from build123d import *

# Parameters (mm, degrees)
F0_W     = 1.7
F0_H     = 14.3
F3_D     = 11
F3_DEPTH = 80
F3_TIP   = 3.3047334047
F5_D     = 11
F5_DEPTH = 80
F5_TIP   = 3.3047334047


with BuildPart() as f1:
    # F0 (on Front) → F1 (revolve)
    with BuildSketch(Plane.XZ):
        Polygon((534, 14.3), (534, 0), (540, 0), (540, 15), (534, 15), align=None)
        with Locations((533.15, 7.15)):
            Rectangle(F0_W, F0_H)
        Polygon((0, 15), (0, 0), (532.3, 0), (532.3, 14.3), (532.3, 15), align=None)
        Polygon((-532.3, 15), (-532.3, 14.3), (-532.3, 0), (0, 0), (0, 15), align=None)
        with Locations((-533.15, 7.15)):
            Rectangle(F0_W, F0_H)
        Polygon((-534, 15), (-540, 15), (-540, 0), (-534, 0), (-534, 14.3), align=None)
    revolve(axis=Axis((-281.0423572082, 0, 0), (-1, 0, 0)))

    # F3
    with Locations(Plane(origin=(-540, 0, 0), x_dir=(0, -1, 0), z_dir=(-1, 0, 0))):
        with Locations((0, 0)):
            Hole(F3_D / 2, depth=F3_DEPTH)
            with Locations((0, 0, -(F3_DEPTH + F3_TIP / 2))):  # 118° drill point
                Cone(0, F3_D / 2, F3_TIP, mode=Mode.SUBTRACT)

    # F5
    with Locations(Plane.YZ.offset(540)):
        with Locations((0, 0)):
            Hole(F5_D / 2, depth=F5_DEPTH)
            with Locations((0, 0, -(F5_DEPTH + F5_TIP / 2))):  # 118° drill point
                Cone(0, F5_D / 2, F5_TIP, mode=Mode.SUBTRACT)


solid = f1.part
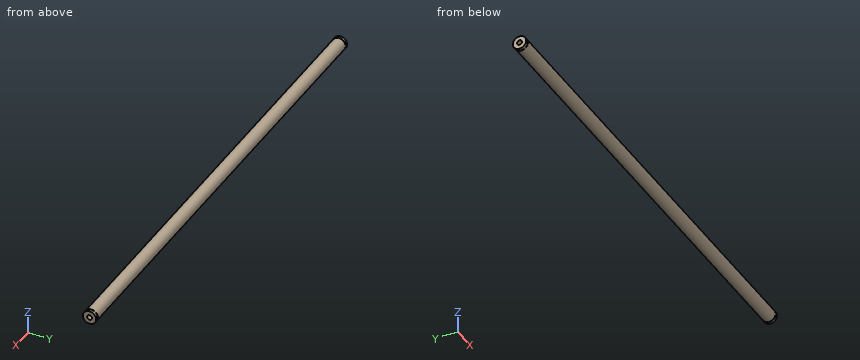
Can you work these out from the model? Positions are in its coordinate system, mm. Give positions to 0.01 mm unless a question says otherwise; leave off trailing zeros. Loops run counter-clockwise (first coordinate to the right, second up) from the corner with the lowest first, then second, coordinate; pieces in that order, holes last. Notation, with made-up numbers: (-1, -1.5) - (26, -1.5) arc R20 ccw to (26, 2.5) - close; hole circle Ø11 at (62.25, 71.5). An arc over 180 degrees is marked (long way). One line per item, written item: value.
(1) I'm going to push flat-ended pins straight in: pin 1 (6 mm diameter, centred on x = -19.5, z = -9.5, fed in from +Y); pin 2 (12 mm diameter, centred on x = -101, y = -8.5, fed in from +Z); pin 3 (10 mm diameter, centred on x = -267.5, z = 5.5, fed in from -Y); pin 4 (9 mm diameter, centred on y = -1.5, z = -4, fed in from +X). Where does each tip first touch, or does it pass through?
Verdict:
pin 1: y = 13.52
pin 2: z = 14.79
pin 3: y = -14.99
pin 4: x = 540
(2) If we section it at A-A, the plane x = 68.5: List the corners of the cut face in (y, z) for me, plus the area to 3 significant figures.
Verdict:
outline: circle Ø30 at (0, 0)
area: 707 mm^2
(3) I need wall thicknesses on line 1 along X through (y, z) = (13.25, 6.5); line 2 along Y through (x, z) = (-492, 0); line 3 along Y through (x, z) = (-15, 1.25). Which ranges of each line are inside material? Lowest first, please.
Verdict:
line 1: -540 to -534, -532.3 to 532.3, 534 to 540
line 2: -15 to -5.5, 5.5 to 15
line 3: -14.95 to 14.95
